from build123d import *

# Parameters (mm, degrees)
SKETCH1_W           = 64.516
SKETCH1_H           = 119.888
BOSS_EXTRUDE1_DEPTH = 28.067
SKETCH2_W           = 58.42
SKETCH2_H           = 113.792
CUT_EXTRUDE1_DEPTH  = 23.2156
SKETCH3_W           = 56.896
SKETCH3_H           = 3.048
CUT_EXTRUDE2_DEPTH  = 23.2156


with BuildPart() as part:
    # Sketch1 → Boss-Extrude1 (new body)
    with BuildSketch(Plane(origin=(0, 0, 0), x_dir=(1, 0, 0), z_dir=(0, 1, 0))):
        with Locations((32.258, 59.944)):
            Rectangle(SKETCH1_W, SKETCH1_H)
    extrude(amount=BOSS_EXTRUDE1_DEPTH)

    # Sketch2 → Cut-Extrude1 (cut)
    with BuildSketch(Plane(origin=(0, 28.067, 0), x_dir=(1, 0, 0), z_dir=(0, 1, 0))):
        with Locations((32.258, 59.944)):
            Rectangle(SKETCH2_W, SKETCH2_H)
    extrude(amount=-CUT_EXTRUDE1_DEPTH, mode=Mode.SUBTRACT)

    # Sketch3 → Cut-Extrude2 (cut)
    with BuildSketch(Plane(origin=(0, 28.067, 0), x_dir=(1, 0, 0), z_dir=(0, 1, 0))):
        with Locations((32.258, 118.364)):
            Rectangle(SKETCH3_W, SKETCH3_H)
        with Locations((32.258, 1.524)):
            Rectangle(SKETCH3_W, SKETCH3_H)
    extrude(amount=-CUT_EXTRUDE2_DEPTH, mode=Mode.SUBTRACT)


solid = part.part
Work out the finished part from the listing and answer in its coordinate system (mm). A direction names the side the tool comes from. Give positions to 0.01 mm unless a question says otherwise; leave off trailing zeros. Order: outer loops, then holes, each group sorted by start corner. A loop starts at its lowest first (then second) coordinate and runs counter-clockwise, first axis right, second up. Notation, with made-up numbers: (-22.75, 33.25) -> (33.25, 33.25) arc R15 ccw to (33.25, 48.25) -> close; hole circle Ø6 at (88, -4). An arc over 180 degrees is marked (long way). Answer as a JSON object with one key per item and string values. Group by question number.
1. The mould has two halves that part along Z. Classify faces 4 (the flat face through (32.1, 4.6, 0)), 5 (the flat face through (3.81, 17, -118)), 6 (the flat face through (61.468, 17, -59)), 7 (the flat face through (32.1, 4.6, -119.888)): released by +Z, released by -Z, zero draft, split by the parting line, or undercut.
2. Section B-B on z = -100 is taken. Determine the outline of the cut face in (x, y).
3. A tool of negligible diameter and unlimited length cuts with its end or side. For faces 1 (the flat face through (3.048, 17, -59)), 2 (the flat face through (60.706, 17, -118)), 3 (the flat face through (63, 28.067, -61)), from which of +Z, -Z, +X, -X, +Y, -Y can it reach the whole face along a straight path? Write none if from no direction.
4. Flat-ended cylindrical pins translate along their axes: pin 1 Ø6 at (x, y) = (9, 16.5) entering from -Z; pin 2 Ø12 at (x, z) = (36, -102) entering from +Y. Find the tip coordinate at first contact, or state that the pin passes through.
5. Section A-A on y = 6.25 is taken. Determine the outline of the cut face in (x, z).
6. Section C-C on x = 46.5 is taken. Determine the outline of the cut face in (y, z).
7. Consider line 1 along X through (y, z) = (26.5, -17.5); line 2 along Y through (x, z) = (61, -98). Determine where each line is inside the solid, lowest interval first. Write a range as [from, to].
Result sheet:
{
 "1": {"face 4": "released by +Z", "face 5": "zero draft", "face 6": "undercut", "face 7": "released by -Z"},
 "2": {"outline": "(0, 0) -> (64.52, 0) -> (64.52, 28.07) -> (61.47, 28.07) -> (61.47, 4.85) -> (3.05, 4.85) -> (3.05, 28.07) -> (0, 28.07) -> close"},
 "3": {"face 1": "+Y", "face 2": "+Z, -Z, +Y", "face 3": "+Z, -Z, +X, -X, +Y"},
 "4": {"pin 1": "passes through", "pin 2": "stops at y = 4.85"},
 "5": {"outline": "(0, -119.89) -> (3.81, -119.89) -> (3.81, -116.84) -> (3.05, -116.84) -> (3.05, -3.05) -> (3.81, -3.05) -> (3.81, 0) -> (0, 0) -> close; (60.71, -119.89) -> (64.52, -119.89) -> (64.52, 0) -> (60.71, 0) -> (60.71, -3.05) -> (61.47, -3.05) -> (61.47, -116.84) -> (60.71, -116.84) -> close"},
 "6": {"outline": "(0, -119.89) -> (4.85, -119.89) -> (4.85, 0) -> (0, 0) -> close"},
 "7": {"line 1": "x = [0, 3.05], [61.47, 64.52]", "line 2": "y = [0, 4.85]"}
}
